```python
from build123d import *

# Parameters (mm, degrees)
BOSS_EXTRUDE1_DEPTH = 6.35
FILLET2_R           = 1.27
SKETCH2_R           = 6.35
CUT_EXTRUDE1_DEPTH  = 7.35


with BuildPart() as part:
    # Sketch1 → Boss-Extrude1 (new body)
    with BuildSketch(Plane(origin=(0, 0, 0), x_dir=(1, 0, 0), z_dir=(0, 1, 0))):
        with BuildLine():
            Line((-25.4, -10.16), (-12.7, -10.16))
            Line((-12.7, -10.16), (-12.7, 0))
            Line((-12.7, 0), (12.7, 0))
            Line((12.7, 0), (12.7, -10.16))
            Line((12.7, -10.16), (25.4, -10.16))
            Line((25.4, -10.16), (25.4, 0))
            ThreePointArc((25.4, 0), (0, 25.4), (-25.4, 0))
            Line((-25.4, 0), (-25.4, -10.16))
        make_face()
    extrude(amount=BOSS_EXTRUDE1_DEPTH)

    # Fillet2
    fillet2_edges = [part.edges().sort_by_distance(p)[0] for p in [
        (-25.4, 0, 5.08),
        (0, 0, -25.4),
        (25.4, 6.35, 5.08),
        (0, 6.35, -25.4),
        (-25.4, 6.35, 5.08),
        (25.4, 0, 5.08),
    ]]
    fillet(fillet2_edges, radius=FILLET2_R)

    # Sketch2 → Cut-Extrude1 (cut, through all)
    with BuildSketch(Plane(origin=(0, 6.35, 0), x_dir=(1, 0, 0), z_dir=(0, 1, 0))):
        with Locations((0, 13.796082309)):
            Circle(SKETCH2_R)
    extrude(amount=-CUT_EXTRUDE1_DEPTH, mode=Mode.SUBTRACT)


solid = part.part
```
Verification items for the finished model (mm, model axes). A direction names the side the tool comes from. Round coordinates to 2 decimals unless told otherwise and drop trailing zeros. Write each loop counter-clockwise with the first axis right and the second up, starting at its lowest first coordinate (ties: lowest second). Pieces come first, ordered by that corner, then holes. Notation, with made-up numbers: (40.25, 39) - (81.25, 39) arc R28 ccw to (81.25, 74) - close; hole circle Ø9 at (-7, 0). An arc over 180 degrees is marked (long way). Answer as a JSON object with one key per item and string values. Group by question number.
Q1. Section check A-A, the plane x = 0. Enter the section's corners in (y, z).
Q2. Tool access check on faces 1 (the flat face through (12.7, 3, 5)), 2 (the cylindrical face through (-25.038, 5.968, 5.151)). Record the directions out of +Z, -Z, +X, -X, +Y, -Y that give a thin tool (end or side, any length) a straight path to the whole face; none if there is none.
Q3. Section check C-C, the plane y = 5.75. Enter the section's corners in (x, z).
Q4. Mould release check, pull along X, two halves, no side actions. Record for faces 3 (the flat face through (0, 3, 0)), 4 (the cylindrical face through (25.038, 0.382, 5.009)), 5 (the flat face through (-19, 3, 10.16)), 6 (the flat face through (-25.4, 3, 5)): released by +X, released by -X, zero draft, split by the parting line, or undercut.
Q5. Section check B-B, the plane z = 4.5. Enter the section's corners in (x, y).
Q6. Go/stop test with flat-tipped pins: pin 1 Ø3 at (y, z) = (5, -15.5) entering from -X; pin 2 Ø1.5 at (x, y) = (-6, 4.5) entering from +Z. Record where each tip stops, or that it passes through.
Q7. Thickness scan on line 1 (Z direction, x = 0, y = 4.5); line 2 (X direction, y = 3.25, z = 7.5); line 3 (X direction, y = 2.5, z = -8.5). Record the ranges inside material, lowest first.
Found:
{
 "1": {"outline": "(0, -24.13) arc R1.27 ccw to (1.27, -25.4) - (5.08, -25.4) arc R1.27 ccw to (6.35, -24.13) - (6.35, -20.15) - (0, -20.15) - close; (0, -7.45) - (6.35, -7.45) - (6.35, 0) - (0, 0) - close"},
 "2": {"face 1": "+Z, +Y, -Y", "face 2": "+Z, -Z, -X, +Y"},
 "3": {"outline": "(-25.21, 0) arc R25.21 ccw to (25.21, 0) - (25.21, 10.16) - (12.7, 10.16) - (12.7, 0) - (-12.7, 0) - (-12.7, 10.16) - (-25.21, 10.16) - close; hole circle Ø12.7 at (0, -13.8)"},
 "4": {"face 3": "undercut", "face 4": "released by +X", "face 5": "zero draft", "face 6": "released by -X"},
 "5": {"outline": "(-25.4, 1.27) arc R1.27 ccw to (-24.13, 0) - (-12.7, 0) - (-12.7, 6.35) - (-24.13, 6.35) arc R1.27 ccw to (-25.4, 5.08) - close; (12.7, 0) - (24.13, 0) arc R1.27 ccw to (25.4, 1.27) - (25.4, 5.08) arc R1.27 ccw to (24.13, 6.35) - (12.7, 6.35) - close"},
 "6": {"pin 1": "stops at x = -21.19", "pin 2": "stops at z = 0"},
 "7": {"line 1": "z = -25.4 to -20.15, -7.45 to 0", "line 2": "x = -25.4 to -12.7, 12.7 to 25.4", "line 3": "x = -23.94 to -3.5, 3.5 to 23.94"}
}
